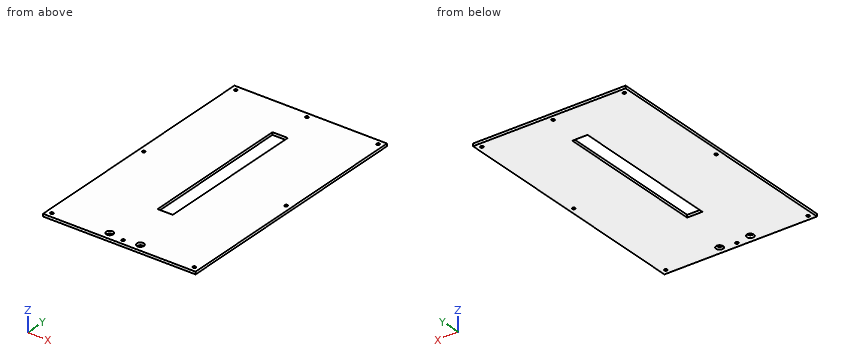
```python
from build123d import *

# Parameters (mm, degrees)
SKETCH1_W           = 300
SKETCH1_H           = 500
SKETCH1_R           = 3
SKETCH1_R_2         = 7
SKETCH1_W_2         = 30
SKETCH1_H_2         = 300
BOSS_EXTRUDE1_DEPTH = 5


with BuildPart() as part:
    # Sketch1 → Boss-Extrude1 (new body)
    with BuildSketch(Plane.XY):
        with Locations((0, -75)):
            Rectangle(SKETCH1_W, SKETCH1_H)
        with Locations((-140, -75)):
            Circle(SKETCH1_R, mode=Mode.SUBTRACT)
        with Locations((140, -315)):
            Circle(SKETCH1_R, mode=Mode.SUBTRACT)
        with Locations((140, -75)):
            Circle(SKETCH1_R, mode=Mode.SUBTRACT)
        with Locations((140, 165)):
            Circle(SKETCH1_R, mode=Mode.SUBTRACT)
        with Locations((0, 165)):
            Circle(SKETCH1_R, mode=Mode.SUBTRACT)
        with Locations((0, -315)):
            Circle(SKETCH1_R, mode=Mode.SUBTRACT)
        with Locations((-140, 165)):
            Circle(SKETCH1_R, mode=Mode.SUBTRACT)
        with Locations((-140, -315)):
            Circle(SKETCH1_R, mode=Mode.SUBTRACT)
        with Locations((-30.15, -310)):
            Circle(SKETCH1_R_2, mode=Mode.SUBTRACT)
        with Locations((30.15, -310)):
            Circle(SKETCH1_R_2, mode=Mode.SUBTRACT)
        with Locations((0, -55)):
            Rectangle(SKETCH1_W_2, SKETCH1_H_2, mode=Mode.SUBTRACT)
    extrude(amount=BOSS_EXTRUDE1_DEPTH)


solid = part.part
```
The model under review builds one solid part; all positions refer to its coordinate system, in mm. Round coordinates to 2 decimals unless told otherwise and drop trailing zeros. Order: outer loops, then holes, each group sorted by start corner. A loop starts at its lowest first (then second) coordinate and runs counter-clockwise, first axis right, second up. Notation, with made-up numbers: (-24, -9.5) -> (10, -9.5) arc R12 ccw to (10, 8.5) -> close; hole circle Ø4 at (1, -29). An arc over 180 degrees is marked (long way). Use a Markdown table: item, result.
Q1. We need section A-A on x = 10. Write out the cut boundary in (y, z).
Values:
| item | result |
|---|---|
| outline | (-325, 0) -> (-205, 0) -> (-205, 5) -> (-325, 5) -> close; (95, 0) -> (175, 0) -> (175, 5) -> (95, 5) -> close |
Q2. We need section C-C on z = 2.1. State how many separate pieces and enclosed holes the cut face has, then the cut area to 3 significant figures.
Values:
| item | result |
|---|---|
| separate pieces | 1 |
| enclosed holes | 11 |
| area | 140,000 mm^2 |
Q3. We need section B-B on y = -86. Write out the cut boundary in (x, z).
Values:
| item | result |
|---|---|
| outline | (-150, 0) -> (-15, 0) -> (-15, 5) -> (-150, 5) -> close; (15, 0) -> (150, 0) -> (150, 5) -> (15, 5) -> close |
Q4. For line 1 (X direction, y = 165, z = 2.55); line 2 (Y direction, x = -140, z = 1.4); line 3 (X direction, y = -310, z = 1.9), list the stretches that pass through material, from the lowest coordinate up.
Values:
| item | result |
|---|---|
| line 1 | x = -150 to -143, -137 to -3, 3 to 137, 143 to 150 |
| line 2 | y = -325 to -318, -312 to -78, -72 to 162, 168 to 175 |
| line 3 | x = -150 to -37.15, -23.15 to 23.15, 37.15 to 150 |
